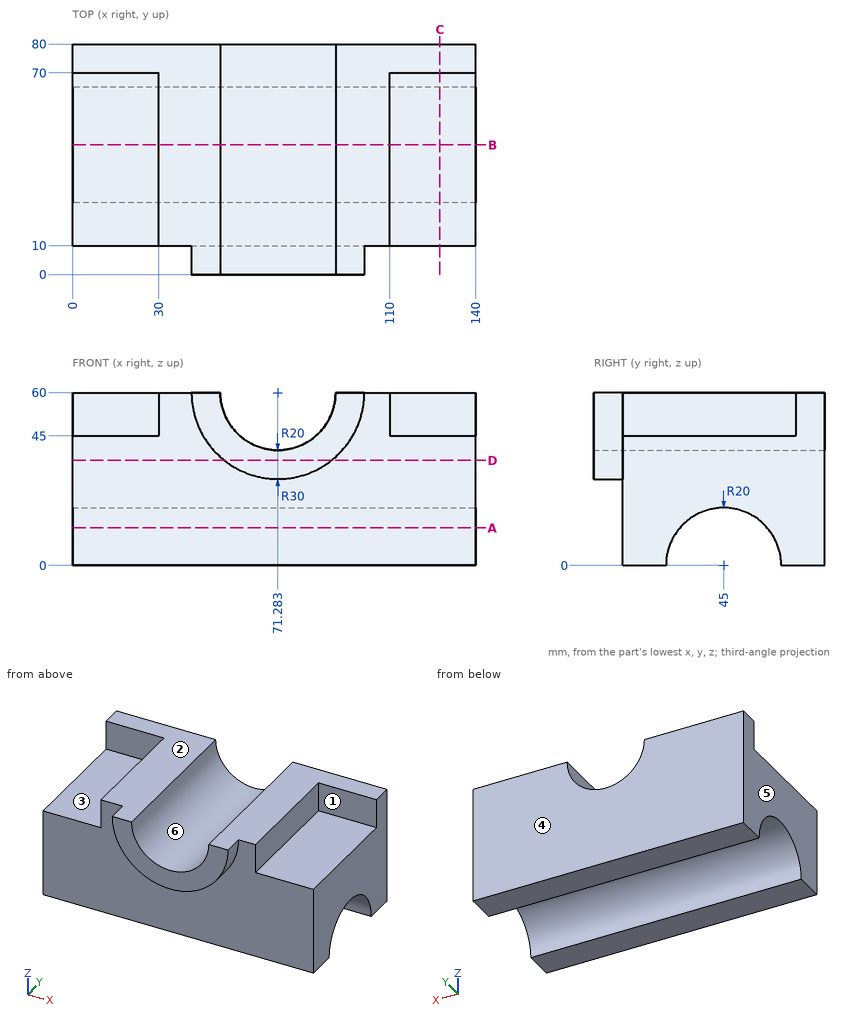
Can you work these out from the drawing? Everything is in mm from the part's minimum corner. A direction names the side the tool comes from. Give positions to 0.01 mm unless a question says otherwise; leave off trailing zeros. Order: outer loops, then holes, each group sorted by start corner. A loop starts at its lowest first (then second) coordinate and runs counter-clockwise, first axis right, second up. Notation, with made-up numbers: M 65,-12.75 L 79,-12.75 A19 ccw 79,15.25 Z; hole C 15.5,29 d1. An arc over 180 degrees is marked long. One line per item, written item: value.
Item 1: Please list where these lines run through material, in increasing order: line 1 (Y direction, x = 90.5, z = 29); line 2 (Z direction, x = 11.5, y = 11); line 3 (Y direction, x = 130, z = 5) (1 decimal).
Verdict:
line 1: 10 to 80
line 2: 0 to 45
line 3: 10 to 25.6, 64.4 to 80
Item 2: For the marked faces 1, 2 and 3, which set-ups out of +Z, -Z, +X, -X, +Y, -Y let a thin tool reach every point of the face, with its end or its side?
Verdict:
face 1: +Z, +X, -Y
face 2: +Z, +X, -X, +Y, -Y
face 3: +Z, -X, -Y
Item 3: For pin 1 (4.5 mm diameter, centred on y = 47.5, z = 55, fed in from -X); pin 2 (4 mm diameter, centred on x = 98.5, z = 38, fed in from -Y); pin 3 (1 mm diameter, centred on x = 48, y = 50.5, fed in from -Z); pin 4 (16.5 mm diameter, centred on y = 53.5, z = 50, fed in from +X), each with a flat end and sliding along its axis, tell me the tip position at first contact or that it passes through.
Verdict:
pin 1: x = 30
pin 2: y = 10
pin 3: z = 19.08
pin 4: x = 140
Item 4: If we section it at C-C on x = 127.5: Write out the boundary of the cut face in (y, z), and give its area (3 significant figures).
Verdict:
outline: M 10,0 L 25,0 A20 cw 65,0 L 80,0 L 80,60 L 70,60 L 70,45 L 10,45 Z
area: 2,670 mm2
Item 5: If we section it at D-D on z = 36.5: Write out the boundary of the cut face in (x, y) (1 decimal).
Verdict:
outline: M 0,10 L 52.6,10 L 52.6,0 L 89.9,0 L 89.9,10 L 140,10 L 140,80 L 0,80 Z
Item 6: If we mould it in two halves opening along X, with no side actions, what happens to the marked faces 4, 5 and 6? For each: pulls with the +X half, pulls with the -X half, needs draft (parallel to the pull), parting line crosses it, or undercut.
Verdict:
face 4: needs draft
face 5: pulls with the -X half
face 6: undercut
Item 7: If we section it at A-A on z = 13: Write out the boundary of the cut face in (x, y), and give its area (3 significant figures).
Verdict:
outline: M 0,10 L 140,10 L 140,29.8 L 0,29.8 Z; M 0,60.2 L 140,60.2 L 140,80 L 0,80 Z
area: 5,540 mm2
Item 8: If we section it at B-B on y = 45: Write out the boundary of the cut face in (x, z).
Verdict:
outline: M 0,20 L 140,20 L 140,45 L 110,45 L 110,60 L 91.28,60 A20 cw 51.28,60 L 30,60 L 30,45 L 0,45 Z
